Read the model definition and answer for the solid it produces. Units are mm, in the model's axes. A direction names the side the tool comes from. Give positions to 0.01 mm unless a question says otherwise; leave off trailing zeros. Write each loop counter-clockwise with the first axis right and the second up, starting at its lowest first coordinate (ties: lowest second). Pieces come first, ordered by that corner, then holes. Notation, with made-up numbers: (-7, -26.5) - (7, -26.5) arc R20 ccw to (7, 9.5) - close; hole circle Ø11 at (10, 58). An arc over 180 degrees is marked (long way). Answer as CSV lines item,"result".
Autodesk Inventor part; units mm, degrees
ref_plane "YZ Plane" through (0, 0, 0) normal (1, 0, 0) x (0, 1, 0)
ref_plane "XZ Plane" through (0, 0, 0) normal (0, 1, 0) x (-1, 0, 0)
ref_plane "XY Plane" through (0, 0, 0) normal (0, 0, 1) x (1, 0, 0)
sketch "Эскиз1" plane through (0, 0, 0) normal (0, 0, 1) x (1, 0, 0)
  circle A0 centre (0, 0) radius 30
  circle A1 centre (0, 0) radius 25
  circle A2 centre (0, 0) radius 28
  line L0 (0, 0) -> (28, 0) construction
  line L1 (0, 0) -> (28, 0) construction
  line L2 (0, 28) -> (-5.2, 28)
  line L3 (-5.2, 28) -> (-5.2, 24.4532)
  line L4 (0, 0) -> (19.799, 19.799)
  line L5 (0, 0) -> (28, 0) construction
  line L6 (-0.4901, 1.1812) -> (26.3238, 1.1812) construction
  line L7 (0, 0) -> (-19.799, 19.799)
  line L8 (0, 0) -> (28, 0) construction
  line L9 (-5.2, 24.4532) -> (5.2, 24.4532)
  line L10 (5.2, 24.4532) -> (5.2, 28)
  line L11 (5.2, 28) -> (0, 28)
  point P0 (4.9999, 24.4949)
  point P1 (-19.4504, 20.1415)
  point P2 (-5.2, 27.5129)
  dimension "d0" = 60
  dimension "d1" = 50
  dimension "d2" = 56
  dimension "d5" = 5.2
  dimension "d7" = 45
  dimension "d11" = 135
  dimension "d19" = 10.4
extrude "Выдавливание1" add sketch "Эскиз1" along normal blind 2 contours L9 A1 | L10 A2 L4 A1 | A1 L4 L7 L9 | A1 L3 A2 L10 | A1 L7 A2 L3
sketch "Эскиз2" plane through (0, 0, 2) normal (0, 0, 1) x (1, 0, 0)
  line L0 (-19.799, 19.799) -> (0, 0)
  circle A0 centre (0, 0) radius 25
  line L1 (-5.2, 28) -> (-5.2, 27.5129)
  circle A1 centre (0, 0) radius 28
  arc A2 (19.799, 19.799) -> (-19.799, 19.799) centre (0, 0) ccw
  line L2 (-5.2, 27.5129) -> (-5.2, 24.4532)
  line L3 (0, 0) -> (19.799, 19.799)
  line L4 (19.799, 19.799) -> (17.6777, 17.6777)
  line L5 (-19.799, 19.799) -> (-17.6777, 17.6777)
  line L6 (-5.2, 24.4532) -> (5.2, 24.4532)
  line L7 (5.2, 24.4532) -> (5.2, 27.5129)
  point P0 (4.9999, 24.4949)
  point P1 (4.9874, 27.5522)
  point P2 (0, 28)
  dimension "d20" = 10.4
extrude "Выдавливание2" add sketch "Эскиз2" along normal blind 11.8 contours A1 L2 A0 L0 | A1 L3 A0 L7
fillet "Сопряжение1" radius 1.5 4 edges at (5.2, 27.5129, 7.9) (5.2, 24.4532, 7.9) (-5.2, 27.5129, 7.9) (-5.2, 24.4532, 7.9)
sketch "Эскиз4" plane through (0, 0, 2) normal (0, 0, 1) x (1, 0, 0)
  line L0 (-17.6777, 17.6777) -> (0, 0)
  circle A0 centre (0, 0) radius 10.5
  dimension "d25" = 21
extrude "Выдавливание3" add sketch "Эскиз4" along normal blind 12 and the other way blind 2
sketch "Эскиз3" plane through (0, 0, 2) normal (0, 0, 1) x (1, 0, 0)
  line L0 (0, 28) -> (0, 29)
  line L1 (0, 29) -> (-5, 29)
  line L2 (-5, 29) -> (-5, 19)
  line L3 (-5, 19) -> (5, 19)
  line L4 (0, 29) -> (5, 29)
  line L5 (5, 29) -> (5, 19)
  line L6 (-1.7678, 18.2322) -> (-10, 10)
  line L7 (-19.799, 19.799) -> (-7.4246, 7.4246)
  line L8 (1.7678, 18.2322) -> (10, 10)
  line L9 (7.4246, 7.4246) -> (17.6777, 17.6777)
  line L10 (10, 10) -> (7.8787, 7.8787)
  circle A0 centre (0, 0) radius 11.1421
  line L11 (-10, 10) -> (-7.8787, 7.8787)
  arc A1 (1.7678, 18.2322) -> (-1.7678, 18.2322) centre (0, 16.4645) ccw
  line L12 (-10, 10) -> (-2.9289, 17.0711)
  line L13 (-2.9289, 17.0711) -> (-10, 24.1421)
  line L14 (-10, 24.1421) -> (-17.0711, 17.0711)
  line L15 (-10, 10) -> (-17.0711, 17.0711)
  line L16 (-7.4246, 7.4246) -> (0, 0)
  arc A2 (7.4246, 7.4246) -> (-7.4246, 7.4246) centre (0, 0) ccw
  line L17 (0, 0) -> (7.4246, 7.4246)
  circle A3 centre (0, 0) radius 28
  circle A4 centre (0, 0) radius 25
  line L18 (0, 11.1421) -> (0, 35.3553)
  line L19 (10, 10) -> (27.088, -7.088)
  line L20 (-10, 10) -> (-27.088, -7.088)
  line L21 (27.088, -7.088) -> (-27.088, -7.088)
  line L22 (-17.0711, 17.0711) -> (-21.6622, 12.4799)
  line L23 (-21.6622, 12.4799) -> (-27.1, 7.0422)
  line L24 (10, 10) -> (17.0711, 17.0711)
  line L25 (17.0711, 17.0711) -> (21.6622, 12.4799)
  line L26 (21.6622, 12.4799) -> (12.4799, 21.6622)
  arc A5 (17.6777, 17.6777) -> (6.3208, 24.1878) centre (0, 0) ccw
  dimension "d21" = 1
  dimension "d22" = 5
  dimension "d23" = 10
  dimension "d24" = 10
  dimension "d31" = 3
  dimension "d32" = 2.5
  dimension "d33" = 10
  dimension "d34" = 10
  dimension "d35" = 22.2843
  dimension "d36" = 16.4645
  dimension "d37" = 7.8223
  dimension "d38" = 10
sketch "Эскиз5" plane through (0, 0, 13.8) normal (0, 0, 1) x (1, 0, 0)
  line L0 (-19.799, 19.799) -> (-7.4246, 7.4246)
  line L1 (-19.799, 19.799) -> (-19.0919, 19.0919)
  line L2 (-19.0919, 19.0919) -> (-9.6913, 23.0452)
  arc A0 (-6.3208, 24.1878) -> (-17.6777, 17.6777) centre (0, 0) ccw
  line L3 (17.6777, 17.6777) -> (19.799, 19.799)
  line L4 (19.799, 19.799) -> (19.0919, 19.0919)
  line L5 (19.0919, 19.0919) -> (9.6913, 23.0452)
  arc A1 (17.6777, 17.6777) -> (6.3208, 24.1878) centre (0, 0) ccw
  line L6 (7.4246, 7.4246) -> (17.6777, 17.6777)
  line L7 (19.0919, 19.0919) -> (17.6777, 17.6777)
  line L8 (-19.0919, 19.0919) -> (-17.6777, 17.6777)
  circle A2 centre (0, 0) radius 25
  dimension "d39" = 1
  dimension "d40" = 1
extrude "Выдавливание4" cut sketch "Эскиз5" against normal blind 11.8 contours L2 A0 L0 | A1 L5 L3
fillet "Сопряжение2" radius 0.595 4 edges at (19.799, 19.799, 6.9) (19.0919, 19.0919, 7.9) (-19.799, 19.799, 6.9) (-19.0919, 19.0919, 7.9)
sketch "Эскиз6" plane through (0, 0, 14) normal (0, 0, 1) x (1, 0, 0)
  circle A0 centre (0, 0) radius 1.5
  dimension "d44" = 3
extrude "Выдавливание5" cut sketch "Эскиз6" against normal blind 14
sketch "Эскиз7" plane through (0, 0, 14) normal (0, 0, 1) x (1, 0, 0)
  circle A0 centre (0, 0) radius 1.5
  line L0 (0, 0) -> (-7.2, 0)
  circle A1 centre (-7.2, 0) radius 0.75
  line L1 (-7.2, 0) -> (-7.2, 3.4)
  line L2 (-7.2, 3.4) -> (-7.2, -3.4)
  circle A2 centre (-7.2, 3.4) radius 0.75
  circle A3 centre (-7.2, -3.4) radius 0.75
  dimension "d47" = 7.2
  dimension "d48" = 1.5
  dimension "d49" = 3.4
  dimension "d50" = 6.8
  dimension "d51" = 1.5
  dimension "d52" = 1.5
extrude "Выдавливание6" cut sketch "Эскиз7" against normal blind 14 contours A3 | A2 | A1 L2 L0 | L0 L1 A1 | L2 A1 L1
pattern_circular "Круговой массив1" count 4 over 360 about axis through (0, 0, 14) along (0, 0, -1) of "Выдавливание6"
sketch "Эскиз8" plane through (0, 0, 0) normal (0, 0, -1) x (-1, 0, 0)
  circle A0 centre (0, 0) radius 1.5
  circle A1 centre (0, 0) radius 1.5
  circle A2 centre (0, 0) radius 9
  dimension "d61" = 18
extrude "Выдавливание7" cut sketch "Эскиз8" against normal blind 4
sketch "Эскиз12" plane through (0, 0, 13.8) normal (0, 0, 1) x (1, 0, 0)
  arc A0 (-7.0792, 27.0903) -> (-19.3619, 20.2267) centre (0, 0) ccw
  arc A1 (7.0792, 27.0903) -> (6.3208, 24.1878) centre (6.7, 25.639) ccw
  line L0 (-7.0792, 27.0903) -> (7.0792, 27.0903)
  line L1 (7.0792, 27.0903) -> (7.0792, 24.1878)
  line L2 (7.0792, 24.1878) -> (-7.0792, 24.1878)
  line L3 (-7.0792, 24.1878) -> (-7.0792, 27.0903)
extrude "Выдавливание8" add sketch "Эскиз12" along normal blind 11.8 contours L1 L2 A1 L0 | A1 L2 L3 L0
sketch "Эскиз13" plane through (-6.3208, 27.0903, 13.8) normal (0, 1, 0) x (1, 0, 0)
  line L0 (11.5208, 11.8) -> (11.5208, 0)
  line L1 (11.5208, 0) -> (11.5208, 2.2)
  line L2 (11.5208, 2.2) -> (19.5413, 0)
  line L3 (13.4, 0) -> (25.6826, 0)
  line L4 (11.5208, 0) -> (19.5413, 0)
  line L5 (12.6415, 0) -> (0, 0)
  line L6 (1.1208, 11.8) -> (1.1208, 0)
  line L7 (1.1208, 0) -> (1.1208, 2.2)
  line L8 (1.1208, 2.2) -> (-6.8998, 0)
  line L9 (-13.0411, 0) -> (-0.7585, 0)
  line L10 (1.1208, 0) -> (0, 0)
  line L11 (1.1208, 0) -> (-6.8998, 0)
  line L12 (-0.7585, 11.8) -> (-0.7585, 0)
  line L13 (13.4, -11.8) -> (-0.7585, -11.8)
  line L14 (-0.7585, 0) -> (-0.7585, -11.8)
  line L15 (-0.7585, -11.8) -> (13.4, -11.8)
  line L16 (13.4, 0) -> (13.4, -11.8)
  line L17 (13.4, -11.8) -> (13.4, 0)
  line L18 (13.4, 0) -> (-0.7585, 0)
  point P0 (6.3208, 13.8)
  dimension "d64" = 2.2
extrude "Выдавливание9" cut sketch "Эскиз13" against normal mid plane 11.8
sketch "Эскиз15" plane through (0, 0, 4) normal (0, 0, -1) x (-1, 0, 0)
  circle A0 centre (0, 0) radius 2.1
  circle A1 centre (0, 0) radius 1.5
  dimension "d67" = 4.2
extrude "Выдавливание10" add sketch "Эскиз15" along normal blind 0.2
properties part number "pizza_disk"
(1) Each of these flat-tipped pins is pushed along its axis until it touches: P1, Ø1.2, axis at x = 3.4, y = 7.2, coming from the -Z side; P2, Ø1.7, axis at x = -3.4, y = 7.2, coming from the -Z side; P3, Ø4.5, axis at x = -15.5, y = 23, coming from the +Z side; P4, Ø6, axis at x = 14.5, z = 4.5, coming from the +Y side. Where does it stop, or does it pass through?
Worked out:
P1,"passes through"
P2,"stops at z = 4"
P3,"stops at z = 13.8"
P4,"stops at y = 25.53"
(2) A cutting plane is placed at A-A (z = 5.5). Count the separate pieces of the cut face and the enclosed holes in it, and give its area (3 significant figures).
Worked out:
separate pieces,"3"
enclosed holes,"13"
area,"396 mm^2"
(3) A cutting plane is placed at D-D (y = 14). Write down the section's boundary in (x, z), and give its area (3 significant figures).
Worked out:
outline,"(-14, 0) - (14, 0) - (14, 2) - (-14, 2) - close"
area,"56.0 mm^2"
(4) For faces 1 (the cylindrical face through (-3.856, 7.795, 9.07)), 2 (the flat face through (9.154, 24.389, 12.685)), 3 (the cylindrical face through (1.172, 8.923, 1.972)), 4 (the cylindrical face through (8.003, 23.685, 7.34)), 5 (the flat face through (-16, 22, 13.8)), determine the directions among +Z, -Z, +X, -X, +Y, -Y from which every point of the face is accessible in a straight line to the end or side of a thin tool.
Worked out:
face 1,"+Z, -Z"
face 2,"+Z, +Y"
face 3,"-Z"
face 4,"+Z"
face 5,"+Z, +X, -X, +Y, -Y"
(5) Find the intervals of material crossed by L1, parallel to X at y = 0, z = 10; L2, parallel to Y at x = 3.4, z = 7.5; L3, parallel to X at y = 7.2, z = 6.75, in increasing order.
Worked out:
L1,"x = -10.5 to -7.95, -6.45 to -1.5, 1.5 to 6.45, 7.95 to 10.5"
L2,"y = -9.93 to -7.95, -6.45 to 6.45, 7.95 to 9.93"
L3,"x = -7.64 to -4.15, -2.65 to -0.75, 0.75 to 2.65, 4.15 to 7.64"
(6) The mould has two halves that part along Y. Classify faces 6 (the cylindrical face through (-5.768, 26.815, 7.128)), 7 (the flat face through (0, 13, 0)), 8 (the cylindrical face through (-3.91, -7.75, 9.07)): +Y half, -Y half, draft (parallel to the pull), parting line (faces both ways), or undercut.
Worked out:
face 6,"+Y half"
face 7,"draft"
face 8,"undercut"
(7) A cutting plane is placed at B-B (y = -3.4). Write down the section's boundary in (x, z).
Worked out:
outline,"(-9.93, 0) - (-8.33, 0) - (-8.33, 4) - (-7.95, 4) - (-7.95, 14) - (-9.93, 14) - close; (-6.45, 4) - (6.45, 4) - (6.45, 14) - (-6.45, 14) - close; (7.95, 4) - (8.33, 4) - (8.33, 0) - (9.93, 0) - (9.93, 14) - (7.95, 14) - close"
(8) A cutting plane is placed at C-C (x = -3.4). Write down the section's boundary in (y, z), and give its area (3 significant figures).
Worked out:
outline,"(-9.93, 0) - (-8.33, 0) - (-8.33, 4) - (-7.95, 4) - (-7.95, 14) - (-9.93, 14) - close; (-6.45, 4) - (6.45, 4) - (6.45, 14) - (-6.45, 14) - close; (7.95, 4) - (8.33, 4) - (8.33, 0) - (27.79, 0) - (27.79, 2) - (9.93, 2) - (9.93, 14) - (7.95, 14) - close"
area,"217 mm^2"
